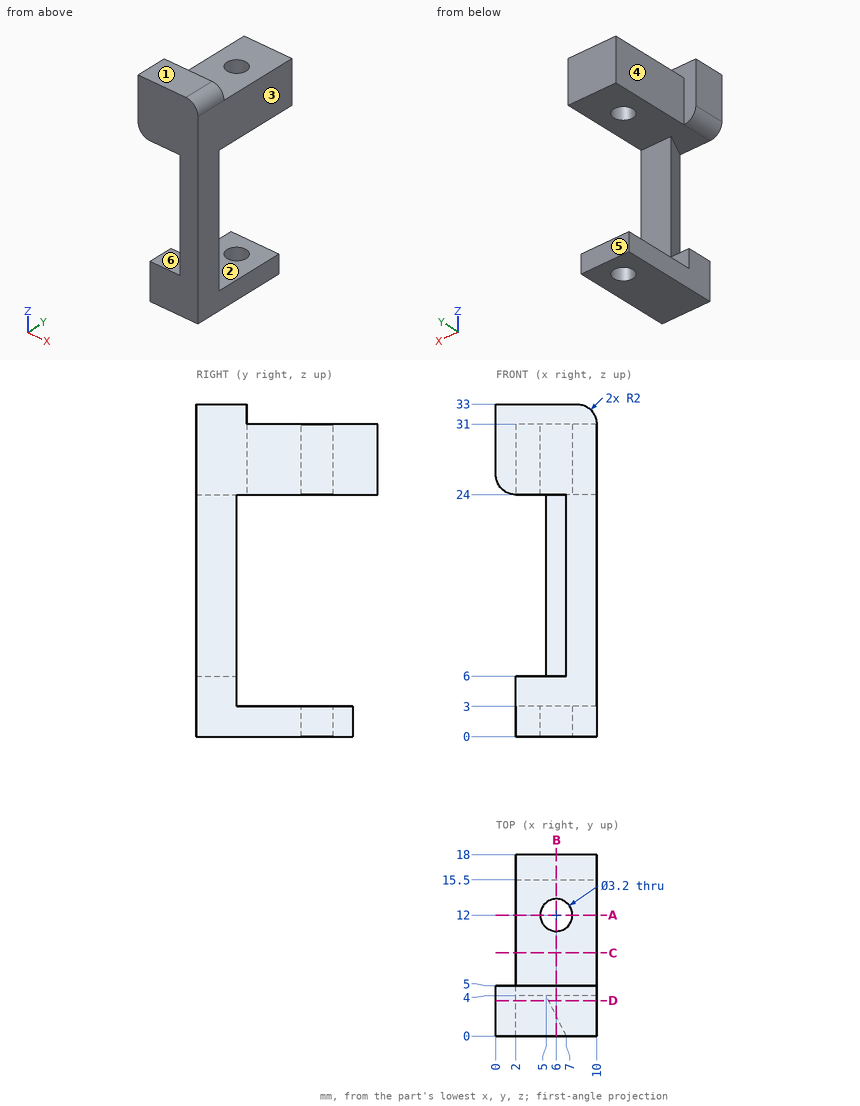
Input: dimensioned drawing with shaded views. Units: mm. Origin: part minimum x, y, z. A direction names the side the tool comes from. Coordinates: 2 decimals unless noted, no trailing zeros. Order: outer loops, then holes, each group sorted by start corner. A loop starts at its lowest first (then second) coordinate and runs counter-clockwise, first axis right, second up.
(1) Section query C-C (y = 8.25). Return the cut outline in (x, z).
(2) Draft query along Z for the marked faces 1, 2 and 3. Return one class per face: pulls with the +Z half, pulls with the -Z half, needs draft (parallel to the pull), parting line crosses it, or undercut.
(3) Material intervals for probe 1 along Z at (x, y) = (4.5, 8); probe 2 along Z at (x, y) = (5, 2.75); probe 3 along Y at (x, z) = (6, 1.4), sorted ascending.
(4) Section query D-D (y = 3.5). Return the cut outline in (x, z), plus the area to 3 significant figures.
(5) Access query for the marked faces 4, 5 and 6. Directions: +Z, -Z, +X, -X, +Y, -Y. A direction counts if a zero-diameter tool reaches every point of the face in a straight line with its end or side. Return the directions, or none.
(6) Section query A-A (y = 12). Return the cut outline in (x, z).
(7) First-contact query: pin 1 (2.5 mm diameter, centred on x = 4, y = 11, fed in from +Z); pin 2 (7.5 mm diameter, centred on y = 13.5, z = 28, fed in from -X); pin 3 (2.5 mm diameter, centred on x = 5.5, z = 2, fed in from +Y). Flat tips, straight axial feed; report the tip coordinate or a pass-through.
(8) Section query B-B (x = 6). Return the cut outline in (y, z).
Solution:
1. outline: (2, 0) - (10, 0) - (10, 3) - (2, 3) - close; (2, 24) - (10, 24) - (10, 31) - (2, 31) - close
2. face 1: pulls with the +Z half
2. face 2: undercut
2. face 3: needs draft
3. probe 1: z = 0 to 3, 24 to 31
3. probe 2: z = 0 to 6, 24 to 33
3. probe 3: y = 0 to 10.4, 13.6 to 15.5
4. outline: (0, 26) arc R2 ccw to (2, 24) - (5.25, 24) - (5.25, 6) - (2, 6) - (2, 0) - (10, 0) - (10, 31) arc R2 ccw to (8, 33) - (0, 33) - close
4. area: 222 mm2
5. face 4: +Z, -Z, -X, +Y
5. face 5: -Z, +X, -X, +Y
5. face 6: -X, -Y
6. outline: (2, 0) - (4.4, 0) - (4.4, 3) - (2, 3) - close; (2, 24) - (4.4, 24) - (4.4, 31) - (2, 31) - close; (7.6, 0) - (10, 0) - (10, 3) - (7.6, 3) - close; (7.6, 24) - (10, 24) - (10, 31) - (7.6, 31) - close
7. pin 1: stops at z = 31
7. pin 2: stops at x = 2
7. pin 3: stops at y = 15.5
8. outline: (0, 0) - (10.4, 0) - (10.4, 3) - (4, 3) - (4, 24) - (10.4, 24) - (10.4, 31) - (5, 31) - (5, 33) - (0, 33) - (0, 24) - (2, 24) - (2, 6) - (0, 6) - close; (13.6, 0) - (15.5, 0) - (15.5, 3) - (13.6, 3) - close; (13.6, 24) - (18, 24) - (18, 31) - (13.6, 31) - close
